Source: CAD feature listing. Evaluate the final solid. Frame: model axes, mm. A direction names the side the tool comes from. Give positions to 0.01 mm unless a question says otherwise; leave off trailing zeros. Order: outer loops, then holes, each group sorted by start corner. A loop starts at its lowest first (then second) coordinate and runs counter-clockwise, first axis right, second up. Notation, with made-up numbers: (40.25, 8.5) - (56.25, 8.5) arc R25 cw to (56.25, 41.5) - close; hole circle Ø8 at (69.5, 41.25). An arc over 180 degrees is marked (long way). One line per item, written item: value. Start each with the question number.
from build123d import *

# Parameters (mm, degrees)
SKETCH1_W                = 10.922
SKETCH1_H                = 17.018
BOSS_EXTRUDE1_DEPTH      = 5.3467
SKETCH2_W                = 12.0015
SKETCH2_H                = 4.4577
CUT_EXTRUDE1_DEPTH       = 9.7536
BOSS_EXTRUDE2_DEPTH      = 10.6934
BOSS_EXTRUDE3_DEPTH      = 9.7536
BOSS_EXTRUDE3_DEPTH_BACK = 8.001
SKETCH4_R                = 3.81


with BuildPart() as part:
    # Sketch1 → Boss-Extrude1 (new, symmetric)
    with BuildSketch(Plane(origin=(0, 0, 0), x_dir=(1, 0, 0), z_dir=(0, 1, 0))):
        Rectangle(SKETCH1_W, SKETCH1_H)
    extrude(amount=BOSS_EXTRUDE1_DEPTH, both=True)

    # Sketch2 → Cut-Extrude1 (cut)
    with BuildSketch(Plane(origin=(5.461, 0, 0), x_dir=(0, 0, -1), z_dir=(1, 0, 0))):
        Rectangle(SKETCH2_W, SKETCH2_H)
    extrude(amount=-CUT_EXTRUDE1_DEPTH, mode=Mode.SUBTRACT)

    # Sketch3 → Boss-Extrude2 (add)
    with BuildSketch(Plane(origin=(0, 5.3467, 0), x_dir=(1, 0, 0), z_dir=(0, 1, 0))):
        with BuildLine():
            Line((-5.461, 8.509), (-5.461, -8.509))
            add(Edge.make_bspline(
                [(-5.461, 8.509), (-46.609, 0), (-5.461, -8.509)],
                knots=[0, 0, 0, 1, 1, 1], degree=2))
        make_face()
    extrude(amount=-BOSS_EXTRUDE2_DEPTH)

    # Sketch4 → Boss-Extrude3 (add, two sides: drawn at the far end of the back side and taken through both)
    with BuildSketch(Plane(origin=(-26.035, 0, 0), x_dir=(0, 0, -1), z_dir=(1, 0, 0)).offset(-BOSS_EXTRUDE3_DEPTH_BACK)):
        Circle(SKETCH4_R)
    extrude(amount=BOSS_EXTRUDE3_DEPTH + BOSS_EXTRUDE3_DEPTH_BACK)


solid = part.part
1. Contact query for flat-ended pins moving along their axis: pin 1 Ø2 at (x, y) = (-10, 2) entering from -Z; pin 2 Ø6 at (x, y) = (-14, 1.5) entering from -Z. Output: stop coordinate, or through.
2. Draft query along Y for faces 3 (the flat face through (0, 0, 8.509)), 4 (the flat face through (1, 0, 6.001)), 5 (the cylindrical face through (-29.41, -1.46, -3.52)). Return one class per face: pulls with the +Y half, pulls with the -Y half, needs draft (parallel to the pull), parting line crosses it, or undercut.
3. Section A-A on x = 3. Return the cut outline in (y, z), then the cut area to 3 significant figures.
4. Set-up query: faces 1 (the flat face through (1, -2.229, 0)), 2 (the flat face through (5.461, 2.5, 0.1)). Return all of +Z, -Z, +X, -X, +Y, -Y with unobstructed straight access to the full face (end or side cutting, diameter ignored); none if empty.
5. Section B-B on x = -27.5. Return the cut outline in (y, z), then the cut area to 3 significant figures.
6. Ray query, L1, parallel to Y at x = 0, z = 0; L2, parallel to X at y = 0.75, z = -2.25; L3, parallel to Y at x = -32, z = 2.75. Return the intervals inside material, ascending.
Data:
1. pin 1: stops at z = -7.74
1. pin 2: stops at z = -7.27
2. face 3: needs draft
2. face 4: undercut
2. face 5: parting line crosses it
3. outline: (-5.35, -8.51) - (5.35, -8.51) - (5.35, 8.51) - (-5.35, 8.51) - close; hole (-2.23, -6) - (2.23, -6) - (2.23, 6) - (-2.23, 6) - close
3. area: 128 mm2
4. face 1: +X
4. face 2: +Z, -Z, +X, +Y, -Y
5. outline: circle Ø7.62 at (0, 0)
5. area: 45.6 mm2
6. L1: y = -5.35 to -2.23, 2.23 to 5.35
6. L2: x = -34.04 to -4.29
6. L3: y = -2.64 to 2.64
